Design review of the part shown in the three views and the two pictorial views. Dimensions are in mm from the part's minimum x, y and z. Coordinates: 2 decimals unless noted, no trailing zeros. Loops run counter-clockwise (first coordinate to the right, second up) from the corner with the lowest first, then second, coordinate; pieces in that order, holes last.
Q1. Add section B-B on x = 25. Give the boundary of the cut face in (y, z).
Q2. Wall thickness on probe 1 along Z at (x, y) = (52, 4.25); probe 2 along X at (y, z) = (13.75, 75); probe 3 along X at (y, z) = (7, 9): over which ranges is each line inside the solid? List them lowest first.
Q3. Add section A-A on z = 75. Give the boundary of the cut face in (x, y).
Q4. For P1, Ø6.5, axis at x = 80, z = 9, coming from the -Y side, flat-tipped, find the tip position at first contact; note if it passes through.
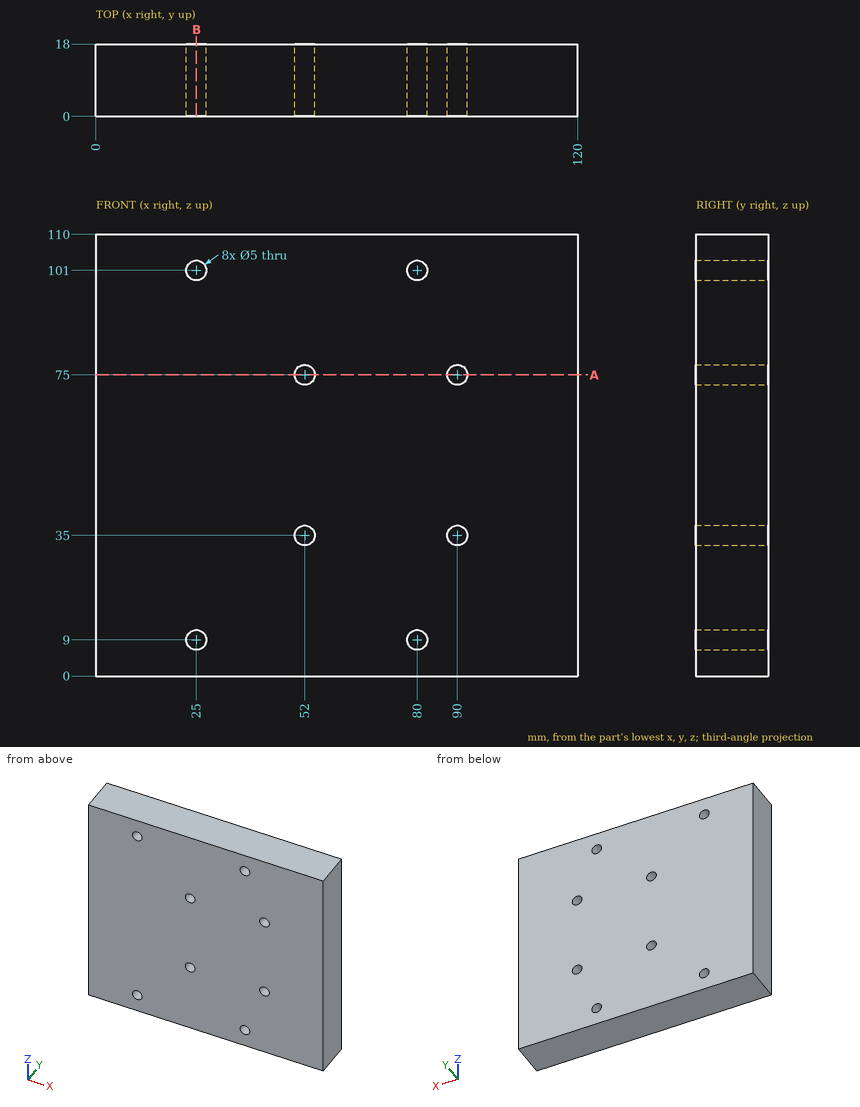
Entries:
1. outline: (0, 0) - (18, 0) - (18, 6.5) - (0, 6.5) - close; (0, 11.5) - (18, 11.5) - (18, 98.5) - (0, 98.5) - close; (0, 103.5) - (18, 103.5) - (18, 110) - (0, 110) - close
2. probe 1: z = 0 to 32.5, 37.5 to 72.5, 77.5 to 110
2. probe 2: x = 0 to 49.5, 54.5 to 87.5, 92.5 to 120
2. probe 3: x = 0 to 22.5, 27.5 to 77.5, 82.5 to 120
3. outline: (0, 0) - (49.5, 0) - (49.5, 18) - (0, 18) - close; (54.5, 0) - (87.5, 0) - (87.5, 18) - (54.5, 18) - close; (92.5, 0) - (120, 0) - (120, 18) - (92.5, 18) - close
4. P1: stops at y = 0
